Read the model definition and answer for the solid it produces. Units are mm, in the model's axes. A direction names the side the tool comes from. Coordinates: 2 decimals unless noted, no trailing zeros. Write each loop counter-clockwise with the first axis right and the second up, starting at its lowest first coordinate (ties: lowest second). Pieces come first, ordered by that corner, then holes. Notation, with made-up numbers: (42.25, 50.5) -> (97.25, 50.5) arc R14 ccw to (97.25, 71.5) -> close; hole circle Ø4 at (86.5, -35). An arc over 180 degrees is marked (long way). Answer as a JSON object with one key per item and string values. Group by question number.
(1) Find section D-D (z = -66.5). Give the vertices of the cut face in (x, y).
(2) Find section A-A (z = 50). Give the vertices of the cut face in (x, y), then the cut area to 3 significant figures.
(3) A flat-ended cylindrical pin translates along its axis: P1, Ø8, axis at x = 28, z = 15, coming from the +Y side. Find the tip coordinate at first contact, or state that the pin passes through.
(4) Straight lines are drawn through the part: L1, parallel to X at y = -4.5, z = 49.5; L2, parallel to Z at x = -65, y = -6.25; L3, parallel to Z at x = 55, y = -1. For each, find the intervals that lie inside material, in ascending order.
(5) Which of the six approach directions +Z, -Z, +X, -X, +Y, -Y give full straight-line access (tool end or side, diameter ignored) to faces 5 (the face through (-49.3, -5.07, -66.547)), 6 (the face through (-1, -10, 1))?
(6) For a pull along X with two mould halves and no side action, classify faces 1 (the face through (53.944, -4.93, 60.138)), 2 (the face through (-1, 0, 1)), 3 (the face through (-66.953, -4.93, 64.872)), 4 (the face through (-100, -5, -1)) as +X half, -X half, draft (parallel to the pull), parting line (faces both ways), or undercut.
(7) Find section B-B (x = -65). Give the vertices of the cut face in (y, z).
(8) Find section C-C (y = -8.5). Give the vertices of the cut face in (x, z).
from build123d import *

# Parameters (mm, degrees)
F0_W     = 200
F0_H     = 170
F0_R     = 15
F1_DEPTH = 10
F3_DEPTH = 10.001


with BuildPart() as f1:
    # F0 (on Front) → F1 (new body)
    with BuildSketch(Plane.XZ):
        Rectangle(F0_W, F0_H)
        with Locations((-65, 50)):
            Circle(F0_R, mode=Mode.SUBTRACT)
        with Locations((65, 50)):
            Circle(F0_R, mode=Mode.SUBTRACT)
    extrude(amount=F1_DEPTH)

    # F2 (on face) → F3 (cut, through all)
    with BuildSketch(Plane.XZ.offset(10)):
        Polygon((0, -48.602977), (-100, -85), (100, -85), align=None)
    extrude(amount=-F3_DEPTH, mode=Mode.SUBTRACT)


solid = f1.part
Results below:
{
 "1": {"outline": "(-100, -10) -> (-49.17, -10) -> (-49.17, 0) -> (-100, 0) -> close; (49.17, -10) -> (100, -10) -> (100, 0) -> (49.17, 0) -> close"},
 "2": {"outline": "(-100, -10) -> (-80, -10) -> (-80, 0) -> (-100, 0) -> close; (-50, -10) -> (50, -10) -> (50, 0) -> (-50, 0) -> close; (80, -10) -> (100, -10) -> (100, 0) -> (80, 0) -> close", "area": "1,400 mm2"},
 "3": {"P1": "stops at y = 0"},
 "4": {"L1": "x = -100 to -79.99, -50.01 to 50.01, 79.99 to 100", "L2": "z = -72.26 to 35, 65 to 85", "L3": "z = -68.62 to 38.82, 61.18 to 85"},
 "5": {"face 5": "-Z, +Y, -Y", "face 6": "+Z, -Z, +X, -X, -Y"},
 "6": {"face 1": "undercut", "face 2": "draft", "face 3": "undercut", "face 4": "-X half"},
 "7": {"outline": "(-10, -72.26) -> (0, -72.26) -> (0, 35) -> (-10, 35) -> close; (-10, 65) -> (0, 65) -> (0, 85) -> (-10, 85) -> close"},
 "8": {"outline": "(-100, -85) -> (0, -48.6) -> (100, -85) -> (100, 85) -> (-100, 85) -> close; hole circle Ø30 at (-65, 50); hole circle Ø30 at (65, 50)"}
}
